Autodesk Inventor part; units mm, degrees
ref_plane "YZ Plane" through (0, 0, 0) normal (1, 0, 0) x (0, 1, 0)
ref_plane "XZ Plane" through (0, 0, 0) normal (0, 1, 0) x (-1, 0, 0)
ref_plane "XY Plane" through (0, 0, 0) normal (0, 0, 1) x (1, 0, 0)
sketch "Sketch1" plane through (0, 0, 0) normal (0, 0, 1) x (1, 0, 0)
  line L0 (-2, 0) -> (20, 0)
  line L1 (20, 0) -> (20, 4)
  line L2 (20, 4) -> (3.125, 4)
  line L3 (3.125, 4) -> (2.3581, 4)
  line L4 (2.3581, 4) -> (0, 4)
  line L5 (0, 4) -> (0, 6.5)
  line L6 (0, 6.5) -> (-8, 6.5)
  line L7 (-8, 6.5) -> (-8, 3.4641)
  line L8 (-8, 3.4641) -> (-4, 3.4641)
  line L9 (-4, 3.4641) -> (-2, 0)
  line L10 (-13.6, 0) -> (25.6, 0)
  line L11 (0, -1.3) -> (0, 7.8)
  line L12 (3.125, 4) -> (0, 4) construction
  dimension "d1" = 16.875
  dimension "d2" = 0.7669
  dimension "d3" = 8
  dimension "d4" = 4
  dimension "d5" = 60
  dimension "d6" = 8
  dimension "d7" = 8
  dimension "d8" = 6.9282
  dimension "d9" = 13
  dimension "d26" = 20
revolve "Body" add sketch "Sketch1" angle 360 about axis through (-2, 0, 0) along (1, 0, 0)
sketch "Sketch2" plane through (-8, 0, 0) normal (-1, 0, 0) x (0, 0, 1)
  circle A0 centre (0, 0) radius 3.4641
  line L0 (0, -9.1) -> (0, 9.1)
  line L1 (-9.1, 0) -> (9.1, 0)
  line L2 (3.4641, 0) -> (1.7321, -3)
  line L3 (1.7321, -3) -> (-1.7321, -3)
  line L4 (-1.7321, -3) -> (-3.4641, 0)
  line L5 (-3.4641, 0) -> (-1.7321, 3)
  line L6 (-1.7321, 3) -> (1.7321, 3)
  line L7 (1.7321, 3) -> (3.4641, 0)
extrude "Slot" add sketch "Sketch2" against normal up to next contours L7 A0 | A0 L2 | L6 L0 A0 | A0 L0 L3 | L0 L6 A0 | A0 L3 L0 | L4 A0 | A0 L5
fillet "Fillet1" radius 0.8 1 edges at (-8, -6.5, 0)
thread "Thread"
equation "\"d1\" = GEL"
equation "\"d3\" = KOH"
equation "\"d4\" = INTI"
equation "\"d6\" = GD"
equation "\"d7\" = BDM"
equation "\"d8\" = 1.1547 * SW"
equation "\"d9\" = KOD"
equation "\"d26\" = NLG"
equation "\"d17\" = RR"
equation "\"d13\" = GEL"
equation "\"GD\" = 8"
equation "\"NLG\" = 20"
equation "\"GEL\" = 16.875"
equation "\"KOD\" = 13"
equation "\"KOH\" = 8"
equation "\"INTI\" = 4"
equation "\"GAL\" = 0.61345 * PTC"
equation "\"GUL\" = 0.61345 * PTC"
equation "\"BDM\" = NND"
equation "\"SW\" = 6"
equation "\"RR\" = 0.8"
equation "\"SPD\" = NND - 1.2269 * PTC"
equation "\"R\" = 0.1"
equation "\"TOA\" = 30deg"
equation "\"GD1\" = THREADDIA - 1.2269 * PTC"
equation "\"THREADDIA\" = 8"
equation "\"FAWI\" = 45deg"
equation "\"PTC\" = 1.25"
equation "\"NND\" = 8"
equation "\"E0\" = 1.155 * SW"
equation "\"d38\" = 55deg"
equation "\"Sketch4_Pitch\" = 1.25"
properties part number "ISO 4762 - M8 x 20" material "Stainless Steel, 440C"
Geometry check sheet. Reference: the model listing, model coordinates, mm. A direction names the side the tool comes from. Round coordinates to 2 decimals unless told otherwise and drop trailing zeros. Order: outer loops, then holes, each group sorted by start corner. A loop starts at its lowest first (then second) coordinate and runs counter-clockwise, first axis right, second up. Notation, with made-up numbers: (1, -25) - (18, -25) arc R20 cw to (18, -1) - close; hole circle Ø9 at (7, -18). An arc over 180 degrees is marked (long way). One line per question, with ' | ' between items. Start each with the question number.
(1) Sectioned sample at A-A on x = -5.5. Record the cut outline in (y, z), and give its area (3 significant figures).
(2) Access from +Z, -Z, +X, -X, +Y, -Y to the whole of each face (thin tool, end or side, straight path). Record for faces 4 (the flat face through (-5.9, -1.5, 2.6)), 5 (the flat face through (20, 0, 0)).
(3) Release check for a two-part mould opening along Z. For faces 1 (the flat face through (0, 3, 3)), 2 (the cylindrical face through (9.86, -0.867, 3.905)), 3 (the flat face through (-6, 3, 0)) record: released by +Z, released by -Z, zero draft, split by the parting line, or undercut.
(4) Thickness scan on L1, parallel to X at y = -3.5, z = 4.5; L2, parallel to Y at x = -4, z = -1.5; L3, parallel to Z at x = 7.25, y = 1. Record the ranges inside material, lowest first. Write a range as [from, to].
(5) Sectioned sample at B-B on x = 12.75. Record the cut outline in (y, z).
(6) Depth check by flat-ended pin: pin 1 Ø1.5 at (y, z) = (-4, 4) entering from +X; pin 2 Ø1.7 at (x, z) = (-7, -1) entering from +Y. Enter the tip coordinate at first touch or a pass-through.
Conclusion:
1) outline: circle Ø13 at (0, 0); hole (-3, -1.73) - (0, -3.46) - (3, -1.73) - (3, 1.73) - (0, 3.46) - (-3, 1.73) - close | area: 102 mm2
2) face 4: -X | face 5: +Z, -Z, +X, +Y, -Y
3) face 1: zero draft | face 2: split by the parting line | face 3: undercut
4) L1: x = [-8, 0] | L2: y = [-6.32, -3], [3, 6.32] | L3: z = [-3.87, 3.87]
5) outline: circle Ø8 at (0, 0)
6) pin 1: stops at x = 0 | pin 2: stops at y = 6.5
